Build history of the part. All positions in model axes, mm. Round coordinates to 2 decimals unless told otherwise and drop trailing zeros. Loops run counter-clockwise (first coordinate to the right, second up) from the corner with the lowest first, then second, coordinate; pieces in that order, holes last.
from build123d import *

# Parameters (mm, degrees)
SKETCH035_R   = 11
SKETCH035_R_2 = 10
PAD013_DEPTH  = 6


with BuildPart() as bearing_outer_front_left:
    # Sketch035 → Pad013 (new body)
    with BuildSketch(Plane.YZ):
        Circle(SKETCH035_R)
        Circle(SKETCH035_R_2, mode=Mode.SUBTRACT)
    extrude(amount=PAD013_DEPTH)


with BuildPart() as bearing_outer_front_left_1:
    # Body007 placement: moved
    add(bearing_outer_front_left.part.moved(Location((6, -51, -44))))


with BuildPart() as bearing_outer_back_left:
    # Part__Mirroring003: instance of bearing-outer-front-left
    add(bearing_outer_front_left_1.part.mirror(Plane(origin=(9, -4e-06, -44.000004), x_dir=(1, 0, 0), z_dir=(0, 1, 0))))


with BuildPart() as bearing_outer_back_right:
    # Part__Mirroring004: instance of bearing-outer-back-left
    add(bearing_outer_back_left.part.mirror(Plane(origin=(-4e-06, 51, -44.000004), x_dir=(0, -1, 0), z_dir=(1, 0, 0))))


solid = bearing_outer_back_right.part
(1) Slice it at B-B on z = -51.25. List the corners of the cut face in (x, y), plus the area to 3 significant figures.
Responses:
outline: (-12, 42.73) - (-6, 42.73) - (-6, 44.11) - (-12, 44.11) - close; (-12, 57.89) - (-6, 57.89) - (-6, 59.27) - (-12, 59.27) - close
area: 16.6 mm2
(2) Pull direction Y, two halves, no side cores. Call faces 1 (the face through (-9, 62, -44)), 2 (the face through (-9, 59, -50)), 3 (the face through (-12, 49, -54)): +Y half, -Y half, draft (parallel to the pull), parting line (faces both ways), or undercut.
Responses:
face 1: parting line
face 2: undercut
face 3: draft
(3) Slice it at C-C on x = -11.6. List the corners of the cut face in (y, z).
Responses:
outline: circle Ø22 at (51, -44); hole circle Ø20 at (51, -44)
(4) Pin check, flat tips, straight feed: P1, Ø6, axis at y = 55.5, z = -41.5, coming from the +X side; P2, Ø1, axis at x = -9, z = -52.5, coming from the +Y side; P3, Ø3, axis at x = -7.5, z = -50.5, coming from the -Y side; P4, Ø1.5, axis at x = -9, y = 43, coming from the +Z side. Stop position of each tip, or through.
Responses:
P1: passes through
P2: stops at y = 58.55
P3: stops at y = 41.2
P4: stops at z = -35.73
(5) Probe line 1 (Z direction, x = -7.55, y = 51); line 2 (Y direction, x = -11.15, z = -36.25); line 3 (Z direction, x = -9.4, y = 44.5). List the from-to ranges inside material, lowest first.
Responses:
line 1: z = -55 to -54, -34 to -33
line 2: y = 43.19 to 44.68, 57.32 to 58.81
line 3: z = -52.87 to -51.6, -36.4 to -35.13
(6) Slice it at A-A on y = 49.5. List the corners of the cut face in (x, z), plus the area to 3 significant figures.
Responses:
outline: (-12, -54.9) - (-6, -54.9) - (-6, -53.89) - (-12, -53.89) - close; (-12, -34.11) - (-6, -34.11) - (-6, -33.1) - (-12, -33.1) - close
area: 12.1 mm2
